Can you work these out from the model? Positions are in its coordinate system, mm. A direction names the side the tool comes from. Give positions to 0.01 mm unless a question says otherwise; leave off trailing zeros. Loops run counter-clockwise (first coordinate to the right, second up) from the corner with the lowest first, then second, coordinate; pieces in that order, holes last.
from build123d import *

# Parameters (mm, degrees)
F1_DEPTH  = 10
F4_DEPTH  = 0.375
F5_W      = 20
F5_H      = 2
F6_DEPTH  = 25
F8_DEPTH  = 2
F9_W      = 10
F9_H      = 10
F10_DEPTH = 50


with BuildPart() as f1:
    # F0 (on Right) → F1 (new body)
    with BuildSketch(Plane.YZ):
        Polygon((-30, 0), (0, 0), (30, 0), (30, 70), (20, 70), (20, 10), (-20, 10), (-20, 70), (-30, 70), align=None)
    extrude(amount=F1_DEPTH)

    # F3 (on offset) → F4 (join, symmetric)
    with BuildSketch(Plane.YZ.offset(5)):
        Polygon((-20, 10), (0, 10), (20, 10), (20, 70), (-20, 70), align=None)
    extrude(amount=F4_DEPTH, both=True)

    # F5 (on face) → F6 (join)
    with BuildSketch(Plane(origin=(0, 0, 0), x_dir=(0, -1, 0), z_dir=(-1, 0, 0))):
        Polygon((-30, 0), (0, 0), (30, 0), (30, 2), (-30, 2), align=None)
        with Locations((40, 1)):
            Rectangle(F5_W, F5_H)
        with Locations((-40, 1)):
            Rectangle(F5_W, F5_H)
    extrude(amount=-F6_DEPTH)

    # F7 (on face) → F8 (join)
    with BuildSketch(Plane(origin=(0, 0, 0), x_dir=(0, -1, 0), z_dir=(-1, 0, 0))):
        Polygon((-50, 2), (-30, 2), (-30, 36), align=None)
        Polygon((30, 2), (50, 2), (30, 36), align=None)
    extrude(amount=-F8_DEPTH)

    # F9 (on face) → F10 (join)
    with BuildSketch(Plane(origin=(0, 0, 0), x_dir=(0, -1, 0), z_dir=(-1, 0, 0))):
        with Locations((-37.8820885718, 5)):
            Rectangle(F9_W, F9_H)
        with Locations((37.8820885718, 5)):
            Rectangle(F9_W, F9_H)
    extrude(amount=F10_DEPTH)

    # F12: F1 across plane


with BuildPart() as f1_1:
    add(f1.part)
    add(f1.part.mirror(Plane.YZ.offset(-50)))


solid = f1_1.part
(1) Suppose I cut it at B-B on z = 44.5. List the corners of the cut face in (x, y) for me (3 decimals), plus the area to 3 significant figures.
Returned:
outline: (-110, -30) - (-100, -30) - (-100, -20) - (-104.625, -20) - (-104.625, 20) - (-100, 20) - (-100, 30) - (-110, 30) - (-110, 20) - (-105.375, 20) - (-105.375, -20) - (-110, -20) - close; (0, -30) - (10, -30) - (10, -20) - (5.375, -20) - (5.375, 20) - (10, 20) - (10, 30) - (0, 30) - (0, 20) - (4.625, 20) - (4.625, -20) - (0, -20) - close
area: 460 mm2
(2) Which directions (+Z, -Z, +X, -X, +Y, -Y) give clear straight access to the entire face, cutting with the end or side of a thin tool? Please do faces 5 (the flat face through (-104.625, 0, 40)), 6 (the flat face through (5, 30, 36)), 7 (the flat face through (8, 0, 10)).
Returned:
face 5: +Z
face 6: +Z, +X, +Y
face 7: +Z, +X
(3) Suppose I cut it at D-D on y = -38.5. List the corners of the cut face in (x, z) for me.
Returned:
outline: (-125, 0) - (25, 0) - (25, 2) - (2, 2) - (2, 21.55) - (0, 21.55) - (0, 10) - (-100, 10) - (-100, 21.55) - (-102, 21.55) - (-102, 2) - (-125, 2) - close
(4) Suppose I cut it at C-C on y = 12.5. List the corners of the cut face in (x, z) for me (3 decimals), plus the area to 3 significant figures.
Returned:
outline: (-125, 0) - (-100, 0) - (-100, 10) - (-104.625, 10) - (-104.625, 70) - (-105.375, 70) - (-105.375, 10) - (-110, 10) - (-110, 2) - (-125, 2) - close; (0, 0) - (25, 0) - (25, 2) - (10, 2) - (10, 10) - (5.375, 10) - (5.375, 70) - (4.625, 70) - (4.625, 10) - (0, 10) - close
area: 350 mm2
(5) Thinking about a two-plate mould opening in X: for faces 1 (the flat face through (2, -20, 40)), 2 (the flat face through (5.375, 0, 40)), 3 (the flat face through (2, 20, 40)), 4 (the flat face through (1, -40, 19)), which applies, pulls with the +X half, pulls with the -X half, needs draft (parallel to the pull), parting line crosses it, or undercut?
Returned:
face 1: undercut
face 2: pulls with the +X half
face 3: undercut
face 4: needs draft
(6) Will these pins go through, and if not, where does the flat tip stop? P1, Ø6, axis at y = -41, z = 12.5, coming from the -X side; P2, Ø5, axis at x = -26, z = 5.5, coming from the -Y side; P3, Ø22, axis at y = 38, z = 14.5, coming from the -X side.
Returned:
P1: stops at x = -102
P2: stops at y = -42.88
P3: stops at x = -110
(7) Please list where these lines run through material, in increasing order: probe 1 along X at (y, z) = (-1, 20.5) (3 decimals); probe 2 along X at (y, z) = (23, 23); probe 3 along Y at (x, z) = (-101.5, 59).
Returned:
probe 1: x = -105.375 to -104.625, 4.625 to 5.375
probe 2: x = -110 to -100, 0 to 10
probe 3: y = -30 to -20, 20 to 30
(8) Suppose I cut it at A-A on x = -78. List the corners of the cut face in (y, z) for me, plus the area to 3 significant figures.
Returned:
outline: (-42.88, 0) - (-32.88, 0) - (-32.88, 10) - (-42.88, 10) - close; (32.88, 0) - (42.88, 0) - (42.88, 10) - (32.88, 10) - close
area: 200 mm2
